CAD build for the part. Positions are in the model's coordinates, mm. Give positions to 0.01 mm unless a question says otherwise; leave off trailing zeros. Write each loop counter-clockwise with the first axis right and the second up, starting at its lowest first coordinate (ties: lowest second). Pieces come first, ordered by that corner, then holes. Notation, with made-up numbers: (-11.5, 8.25) - (45.5, 8.25) arc R15 ccw to (45.5, 25.25) - close; hole circle Ø2 at (-35.75, 62.25). An arc over 180 degrees is marked (long way). Answer as a JSON object with one key per item and string values.
from build123d import *

# Parameters (mm, degrees)
ESQUISSE1_R             = 15
BOSS_EXTRU_1_DEPTH      = 10
ESQUISSE5_R             = 40.5
ESQUISSE5_R_2           = 6
ENL_V_MAT_EXTRU_1_DEPTH = 10
ESQUISSE6_R             = 26
ENL_V_MAT_EXTRU_2_DEPTH = 10
ENL_V_MAT_EXTRU_3_DEPTH = 10
CONG_1_R                = 30
ENL_V_MAT_EXTRU_4_DEPTH = 10


with BuildPart() as part:
    # Esquisse1 → Boss.-Extru.1 (new body)
    with BuildSketch(Plane(origin=(0, 0, 0), x_dir=(0, 0, -1), z_dir=(1, 0, 0))):
        Polygon((540, 0), (540, 310), (195, 310), (0, 150), (0, 0), (0, -10), (110, -10), (110, 0), (210, 0), (210, -10), (330, -10), (330, 0), (430, 0), (430, -10), (540, -10), align=None)
        with Locations((490, 270)):
            Circle(ESQUISSE1_R, mode=Mode.SUBTRACT)
        with Locations((50, 130)):
            Circle(ESQUISSE1_R, mode=Mode.SUBTRACT)
    extrude(amount=BOSS_EXTRU_1_DEPTH)

    # Esquisse5 → Enlèv. mat.-Extru.1 (cut)
    with BuildSketch(Plane.ZY):
        with Locations((-265, 130)):
            Circle(ESQUISSE5_R)
        with Locations((-300.35, 94.65)):
            Circle(ESQUISSE5_R_2)
        with Locations((-300.35, 165.35)):
            Circle(ESQUISSE5_R_2)
        with Locations((-229.65, 165.35)):
            Circle(ESQUISSE5_R_2)
        with Locations((-229.65, 94.65)):
            Circle(ESQUISSE5_R_2)
    extrude(amount=-ENL_V_MAT_EXTRU_1_DEPTH, mode=Mode.SUBTRACT)

    # Esquisse6 → Enlèv. mat.-Extru.2 (cut)
    with BuildSketch(Plane.ZY):
        with Locations((-445, 70)):
            Circle(ESQUISSE6_R)
        with Locations(Location((-85, 70, 0), (0, 0, 180))):
            Circle(ESQUISSE6_R)
    extrude(amount=-ENL_V_MAT_EXTRU_2_DEPTH, mode=Mode.SUBTRACT)

    # Esquisse7 → Enlèv. mat.-Extru.3 (cut)
    with BuildSketch(Plane.ZY):
        Polygon((-198.57749782, 300), (-247.5, 300), (-247.5, 310), (-327.5, 310), (-327.5, 300), (-407.5, 300), (-407.5, 310), (-487.5, 310), (-487.5, 300), (-530, 300), (-530, 280), (-540, 280), (-540, 230), (-530, 230), (-530, 190), (-540, 190), (-540, 140), (-530, 140), (-530, 110), (-794.780536076, 110), (-794.780536076, 495.732813741), (95.631773419, 495.732813741), (95.631773419, 137.064617174), (0, 137.064617174), (-34.266562773, 165.180771244), (-27.923396657, 172.911504949), (-74.307798886, 210.97050165), (-80.650965002, 203.239767945), (-127.035367231, 241.298764646), (-120.692201114, 249.02949835), (-167.076603343, 287.088495051), (-173.41976946, 279.357761346), align=None)
    extrude(amount=-ENL_V_MAT_EXTRU_3_DEPTH, mode=Mode.SUBTRACT)

    # Congé1
    # the kernel refuses this fillet: 30 mm, written as the material it takes off along each edge
    with BuildSketch(Plane(origin=(-75, -10, -540), x_dir=(0, 1, 0), z_dir=(1, 0, 0)), Plane(origin=(-75, -10, 0), x_dir=(0, 0, -1), z_dir=(1, 0, 0))) as cong_1_piece_1:
        with BuildLine():
            CenterArc((CONG_1_R, CONG_1_R), CONG_1_R, 180, 90)
            Line((0, CONG_1_R), (-CONG_1_R * 0.02, CONG_1_R))
            Line((-CONG_1_R * 0.02, CONG_1_R), (-CONG_1_R * 0.02, -CONG_1_R * 0.02))
            Line((-CONG_1_R * 0.02, -CONG_1_R * 0.02), (CONG_1_R, -CONG_1_R * 0.02))
            Line((CONG_1_R, -CONG_1_R * 0.02), (CONG_1_R, 0))
        make_face()
    extrude(amount=160, mode=Mode.SUBTRACT)
    with BuildSketch(Plane(origin=(-70.710678119, 300, -530), x_dir=(0, -1, 0), z_dir=(1, 0, 0))) as cong_1_piece_2:
        with BuildLine():
            CenterArc((30, -28.284271247), CONG_1_R, 109.471220634, 70.528779366)
            Line((0, -28.284271247), (-0.6, -28.284271247))
            Line((-0.6, -28.284271247), (-0.6, 0))
            Line((-0.6, 0), (0, 0.6))
            ThreePointArc((0, 0.6), (10, 0.6), (19.8, 0.565685425))
            Line((19.8, 0.565685425), (20, 0))
        make_face()
    extrude(amount=151.421356237, mode=Mode.SUBTRACT)
    with BuildSketch(Plane(origin=(-35.476909659, 137.064617174, 0), x_dir=(0, -1, 0), z_dir=(1, 0, 0))) as cong_1_piece_3:
        with BuildLine():
            CenterArc((CONG_1_R * 0.473025462116, CONG_1_R), CONG_1_R, 219.369317242, 50.630682758)
            Line((-CONG_1_R * 0.300047908367, CONG_1_R * 0.365683388322), (-CONG_1_R * 0.315509375776, CONG_1_R * 0.352997056088))
            Line((-CONG_1_R * 0.315509375776, CONG_1_R * 0.352997056088), (-CONG_1_R * 0.00946050924232, -CONG_1_R * 0.02))
            Line((-CONG_1_R * 0.00946050924232, -CONG_1_R * 0.02), (CONG_1_R * 0.473025462116, -CONG_1_R * 0.02))
            Line((CONG_1_R * 0.473025462116, -CONG_1_R * 0.02), (CONG_1_R * 0.473025462116, 0))
        make_face()
    extrude(amount=80.953819317, mode=Mode.SUBTRACT)
    with BuildSketch(Plane(origin=(-26.831233647, 300, -198.57749782), x_dir=(0, -0.634316611678022, 0.7730733704825911), z_dir=(1, 0, 0))) as cong_1_piece_4:
        with BuildLine():
            CenterArc((CONG_1_R * 0.357749781954, CONG_1_R), CONG_1_R, 230.630682758, 39.369317242)
            Line((-CONG_1_R * 0.276566829724, CONG_1_R * 0.226926629517), (-CONG_1_R * 0.289253161958, CONG_1_R * 0.211465162108))
            Line((-CONG_1_R * 0.289253161958, CONG_1_R * 0.211465162108), (-CONG_1_R * 0.00715499563907, -CONG_1_R * 0.02))
            Line((-CONG_1_R * 0.00715499563907, -CONG_1_R * 0.02), (CONG_1_R * 0.357749781954, -CONG_1_R * 0.02))
            Line((CONG_1_R * 0.357749781954, -CONG_1_R * 0.02), (CONG_1_R * 0.357749781954, 0))
        make_face()
    extrude(amount=63.662467293, mode=Mode.SUBTRACT)

    # Esquisse8 → Enlèv. mat.-Extru.4 (cut)
    with BuildSketch(Plane.ZY):
        Polygon((-355.35, 210), (-365.35, 220), (-470, 220), (-480, 210), (-480, 140), (-470, 130), (-365.35, 130), (-355.35, 140), align=None)
    extrude(amount=-ENL_V_MAT_EXTRU_4_DEPTH, mode=Mode.SUBTRACT)


solid = part.part
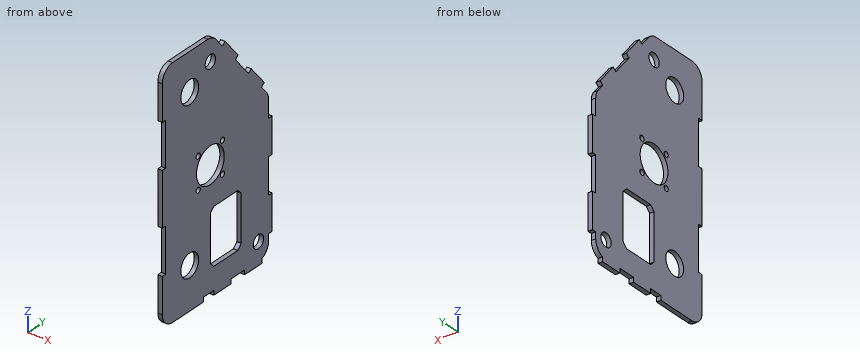
(1) Saw through at A-A, the plane y = 70. Give the cut face in (x, z), and give its area (3 significant figures).
Answer key:
{"outline": "(0, -540) - (10, -540) - (10, -471) - (0, -471) - close; (0, -419) - (10, -419) - (10, -111) - (0, -111) - close; (0, -59) - (10, -59) - (10, 0) - (0, 0) - close", "area": "4,360 mm²"}
(2) Saw through at D-D, the plane x = 2. State how many separate pieces and enclosed holes the cut face has, and give its area (3 significant figures).
Answer key:
{"separate pieces": "1", "enclosed holes": "10", "area": "128,000 mm²"}
(3) Saw through at C-C, the plane y = 183. Give the cut face in (x, z).
Answer key:
{"outline": "(0, -540) - (10, -540) - (10, -480) - (0, -480) - close; (0, -355.35) - (10, -355.35) - (10, -40.22) - (0, -40.22) - close"}
(4) Flat gauge pins, fed straight in: P1, Ø3, axis at x = 7, y = -2.5, coming from the -Z side; P2, Ø3, axis at x = 3.5, z = -376, coming from the -Y side; P3, Ø3, axis at x = 5, z = -532.5, coming from the -Y side; P4, Ø3, axis at y = 86, z = -308, coming from the -X side. Where does each tip first touch, or does it go through?
Answer key:
{"P1": "stops at z = -531.42", "P2": "stops at y = 0", "P3": "stops at y = -1.42", "P4": "stops at x = 0"}
(5) Saw through at B-B, the plane z = -50. Give the cut face in (x, y), and give its area (3 significant figures).
Answer key:
{"outline": "(0, -10) - (10, -10) - (10, 115) - (0, 115) - close; (0, 145) - (10, 145) - (10, 191.03) - (0, 191.03) - close", "area": "1,710 mm²"}
(6) Probe L1, parallel to Z at x = 4.25, y = 69.5; L2, parallel to Y at x = 2, z = -445; L3, parallel to Y at x = 8, z = -300.35. List the from-to ranges inside material, lowest first. Write a range as [from, to].
Answer key:
{"L1": "z = [-540, -471], [-419, -111], [-59, 0]", "L2": "y = [-10, 44], [96, 130], [220, 310]", "L3": "y = [-10, 88.65], [100.65, 110.24], [149.76, 159.35], [171.35, 310]"}
